Input: part model. Units: mm. Frame: model coordinates. Give positions to 0.01 mm unless a question says otherwise; leave off trailing zeros. Write each loop counter-clockwise with the first axis right and the second up, starting at its lowest first coordinate (ties: lowest second). Pieces come first, ordered by that corner, then holes.
```python
from build123d import *

# Parameters (mm, degrees)
F0_W     = 990.6
F0_H     = 38.1
F1_DEPTH = 88.9
F3_DEPTH = 88.901
F5_DEPTH = 88.901


with BuildPart() as f1:
    # F0 (on Front) → F1 (new body)
    with BuildSketch(Plane.XZ):
        Rectangle(F0_W, F0_H)
    extrude(amount=F1_DEPTH)

    # F2 (on face) → F3 (cut, through all)
    with BuildSketch(Plane.XZ.offset(88.9)):
        Polygon((-457.2, -19.05), (-495.3, 19.05), (-495.3, -19.05), align=None)
    extrude(amount=-F3_DEPTH, mode=Mode.SUBTRACT)

    # F4 (on Front) → F5 (cut, through all)
    with BuildSketch(Plane.XZ):
        Polygon((495.3, -19.05), (495.3, 19.05), (457.2, -19.05), align=None)
    extrude(amount=F5_DEPTH, mode=Mode.SUBTRACT)


solid = f1.part
```
Q1. Section A-A, the plane z = 7. Return the cut outline in (x, y).
Q2. Material intervals for line 1 along X through (y, z) = (-55.5, 11); line 2 along X through (y, z) = (-16, 8), sorted ascending.
Q3. Pin query (flat end, axial travel): pin 1 (1 mm diameter, centred on y = -54.5, z = 13.5, fed in from -X); pin 2 (8 mm diameter, centred on x = 58, z = -9, fed in from +Y); pin 3 (4 mm diameter, centred on y = -49, z = 13.5, fed in from -X); pin 4 (1 mm diameter, centred on y = -49, z = 12.5, fed in from +X). Return the tip coordinate at first contact, or that it passes through.
Q4. Section B-B, the plane y = -68. Return the cut outline in (x, z), then the cut area to 3 significant figures.
Solutions:
1. outline: (-483.25, -88.9) - (483.25, -88.9) - (483.25, 0) - (-483.25, 0) - close
2. line 1: x = -487.25 to 487.25
2. line 2: x = -484.25 to 484.25
3. pin 1: stops at x = -490.25
3. pin 2: stops at y = 0
3. pin 3: stops at x = -491.75
3. pin 4: stops at x = 489.25
4. outline: (-495.3, 19.05) - (-457.2, -19.05) - (457.2, -19.05) - (495.3, 19.05) - close
4. area: 36,300 mm2
